```python
from build123d import *

# Parameters (mm, degrees)
SKETCH1_W           = 101.6
SKETCH1_H           = 101.6
BOSS_EXTRUDE1_DEPTH = 3.175
FILLET1_R           = 5
SKETCH2_R           = 3.25
CUT_EXTRUDE1_DEPTH  = 3.175
LPATTERN1_COUNT     = 3
LPATTERN1_PITCH     = 20
LPATTERN2_COUNT     = 3
LPATTERN2_PITCH     = 20


with BuildPart() as part:
    # Sketch1 → Boss-Extrude1 (new body)
    with BuildSketch(Plane(origin=(0, 0, 0), x_dir=(1, 0, 0), z_dir=(0, 1, 0))):
        Rectangle(SKETCH1_W, SKETCH1_H)
    extrude(amount=BOSS_EXTRUDE1_DEPTH)

    # Fillet1
    fillet1_edges = [part.edges().sort_by_distance(p)[0] for p in [
        (50.8, 1.5875, 50.8),
        (-50.8, 1.5875, 50.8),
        (-50.8, 1.5875, -50.8),
        (50.8, 1.5875, -50.8),
    ]]
    fillet(fillet1_edges, radius=FILLET1_R)

    # Sketch2 → Cut-Extrude1 (cut)
    with BuildSketch(Plane(origin=(0, 3.175, 0), x_dir=(1, 0, 0), z_dir=(0, 1, 0))):
        Circle(SKETCH2_R)
        with Locations((20, 0)):
            Circle(SKETCH2_R)
        with Locations((40, 0)):
            Circle(SKETCH2_R)
        with Locations((-20, 0)):
            Circle(SKETCH2_R)
        with Locations((-40, 0)):
            Circle(SKETCH2_R)
    cut_extrude1 = extrude(amount=-CUT_EXTRUDE1_DEPTH, mode=Mode.SUBTRACT)

    # LPattern1: Cut-Extrude1 ×3
    with Locations(*[(0, 0, i * LPATTERN1_PITCH) for i in range(1, LPATTERN1_COUNT)]):
        add(cut_extrude1, mode=Mode.SUBTRACT)

    # LPattern2: Cut-Extrude1 ×3
    with Locations(*[(0, 0, -i * LPATTERN2_PITCH) for i in range(1, LPATTERN2_COUNT)]):
        add(cut_extrude1, mode=Mode.SUBTRACT)


solid = part.part
```
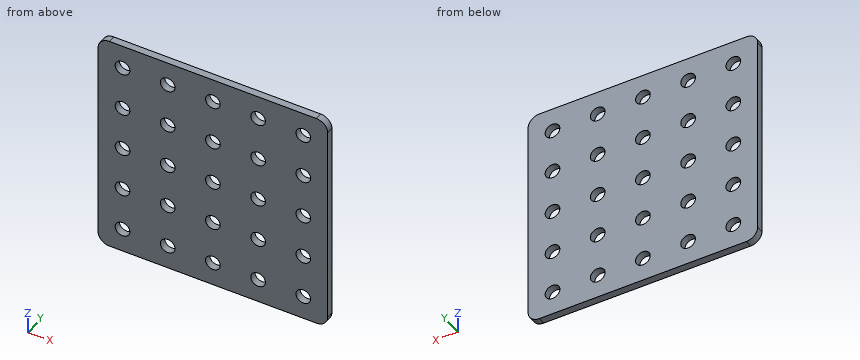
Work out the finished part from the listing and answer in its coordinate system (mm). Give positions to 0.01 mm unless a question says otherwise; leave off trailing zeros. Order: outer loops, then holes, each group sorted by start corner. A loop starts at its lowest first (then second) coordinate and runs counter-clockwise, first axis right, second up.
1. Section C-C, the plane y = 0.6 is taken. Give the number of separate pieces and of enclosed holes in the cut face, and give its area (3 significant figures).
Result sheet:
separate pieces: 1
enclosed holes: 25
area: 9,470 mm2
2. Straight lines are drawn through the part: L1, parallel to Z at x = -40, y = 1.2; L2, parallel to Z at x = -19, y = 0.8. For each, find the intervals that lie inside material, in ascending order.
Result sheet:
L1: z = -50.8 to -43.25, -36.75 to -23.25, -16.75 to -3.25, 3.25 to 16.75, 23.25 to 36.75, 43.25 to 50.8
L2: z = -50.8 to -43.09, -36.91 to -23.09, -16.91 to -3.09, 3.09 to 16.91, 23.09 to 36.91, 43.09 to 50.8
3. Section A-A, the plane x = 0 is taken. Determine the outline of the cut face in (y, z) (3 decimals), and give its area (3 significant figures).
Result sheet:
outline: (0, -50.8) - (3.175, -50.8) - (3.175, -43.25) - (0, -43.25) - close; (0, -36.75) - (3.175, -36.75) - (3.175, -23.25) - (0, -23.25) - close; (0, -16.75) - (3.175, -16.75) - (3.175, -3.25) - (0, -3.25) - close; (0, 3.25) - (3.175, 3.25) - (3.175, 16.75) - (0, 16.75) - close; (0, 23.25) - (3.175, 23.25) - (3.175, 36.75) - (0, 36.75) - close; (0, 43.25) - (3.175, 43.25) - (3.175, 50.8) - (0, 50.8) - close
area: 219 mm2
4. This flat-tipped pin is pushed along its axis until it touches: P1, Ø10.5, axis at x = -20, z = -40, coming from the +Y side (3 decimals). Where does it stop, or does it pass through?
Result sheet:
P1: stops at y = 3.175
5. Section B-B, the plane z = -40 is taken. Determine the outline of the cut face in (x, y) (3 decimals), and give its area (3 significant figures).
Result sheet:
outline: (-50.8, 0) - (-43.25, 0) - (-43.25, 3.175) - (-50.8, 3.175) - close; (-36.75, 0) - (-23.25, 0) - (-23.25, 3.175) - (-36.75, 3.175) - close; (-16.75, 0) - (-3.25, 0) - (-3.25, 3.175) - (-16.75, 3.175) - close; (3.25, 0) - (16.75, 0) - (16.75, 3.175) - (3.25, 3.175) - close; (23.25, 0) - (36.75, 0) - (36.75, 3.175) - (23.25, 3.175) - close; (43.25, 0) - (50.8, 0) - (50.8, 3.175) - (43.25, 3.175) - close
area: 219 mm2
